Source: three-view drawing plus pictorial views. Frame: mm from the lowest corner of the part. A direction names the side the tool comes from. Give positions to 0.01 mm unless a question says otherwise; leave off trailing zeros. Loops run counter-clockwise (first coordinate to the right, second up) from the corner with the lowest first, then second, coordinate; pieces in that order, holes last. Notation, with made-up numbers: (-15.5, -14.5) -> (10.5, -14.5) arc R9 ccw to (10.5, 2.5) -> close; hole circle Ø6 at (75, 81). An arc over 180 degrees is marked (long way). Answer in a Markdown table with one row per item. Add a question column.
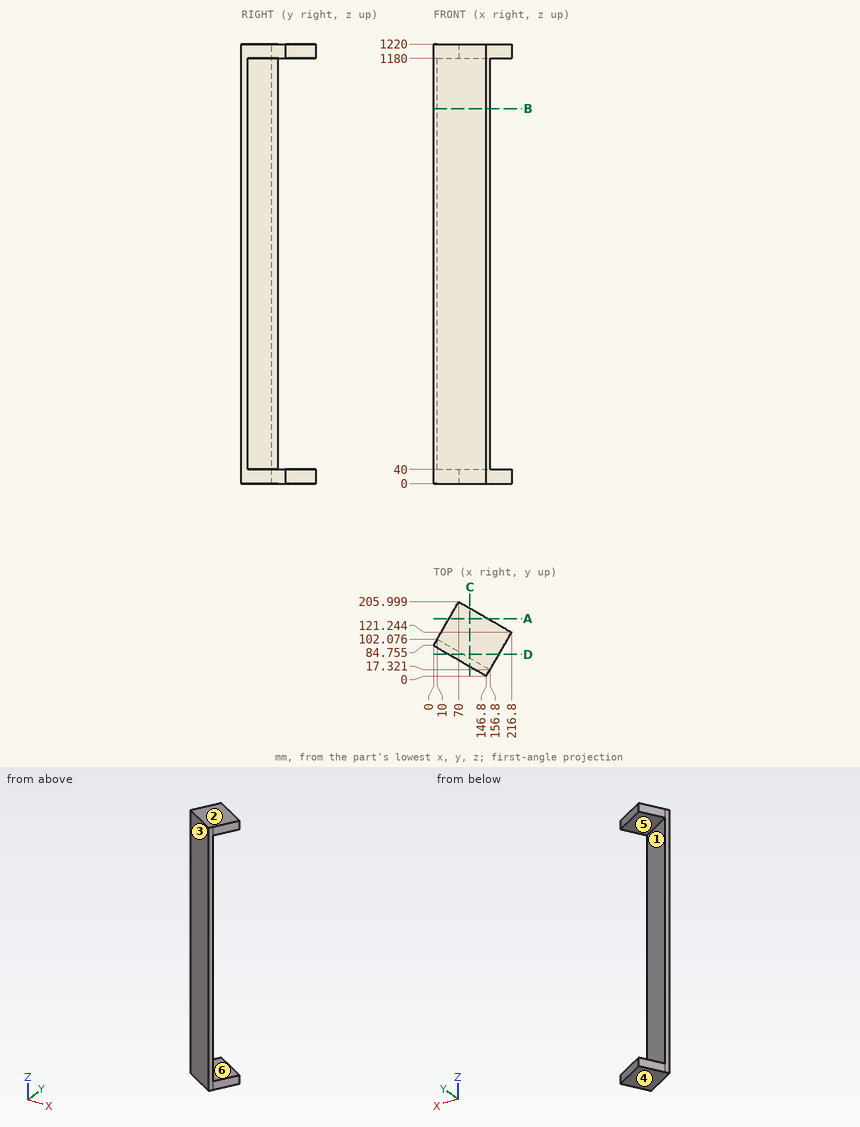
(1) Material intervals for line 1 along Z through (x, y) = (180, 99.5); line 2 along Y through (x, z) = (151, 1076.5) (1 decimal); line 3 along X through (y, z) = (12, 1018.5) (1 decimal), sorted ascending. Write a range as from..to.
(2) Cut plane D-D on y = 60. Return the cut outline in (x, z), then the cut area to 3 significant figures.
(3) Cut plane B-B on z = 1040.5. Return the cut outline in (x, y) (1 decimal), then the cut area to 3 significant figures.
(4) Cut plane A-A on y = 159. Return the cut outline in (x, z) (1 decimal).
(5) Draft query along Z for the marked faces 3, 4, 5 and 6. Return one class per face: +Z half, -Z half, draft (parallel to the pull), parting line (faces both ways), or undercut.
(6) Cut plane C-C on x = 100.5. Return the cut outline in (y, z) (1 decimal).
(7) Pin query (flat end, axial travel): pin 1 Ø1.5 at (x, z) = (54, 790.5) entering from -Y (1 decimal); pin 2 Ø4 at (x, z) = (123, 642.5) entering from -Y (1 decimal); pin 3 Ø10 at (x, z) = (122, 304) entering from +Y. Return the tip coordinate at first contact, or that it passes through.
(8) Reachability of the marked faces 1 and 2 from +Z, -Z, +X, -X, +Y, -Y: full face, straight path, thin tool, end or side. Return the list, or none.
Answer list:
| question | item | result |
|---|---|---|
| 1 | line 1 | z = 0..40, 1180..1220 |
| 1 | line 2 | y = 7.3..20.7 |
| 1 | line 3 | x = 126..153.7 |
| 2 | outline | (42.88, 0) -> (181.44, 0) -> (181.44, 40) -> (82.88, 40) -> (82.88, 1180) -> (181.44, 1180) -> (181.44, 1220) -> (42.88, 1220) -> close |
| 2 | area | 56,700 mm² |
| 3 | outline | (0, 84.8) -> (146.8, 0) -> (156.8, 17.3) -> (10, 102.1) -> close |
| 3 | area | 3,390 mm² |
| 4 | outline | (42.9, 0) -> (151.4, 0) -> (151.4, 40) -> (42.9, 40) -> close; (42.9, 1180) -> (151.4, 1180) -> (151.4, 1220) -> (42.9, 1220) -> close |
| 5 | face 3 | draft |
| 5 | face 4 | -Z half |
| 5 | face 5 | undercut |
| 5 | face 6 | undercut |
| 6 | outline | (26.7, 0) -> (188.4, 0) -> (188.4, 40) -> (49.8, 40) -> (49.8, 1180) -> (188.4, 1180) -> (188.4, 1220) -> (26.7, 1220) -> close |
| 7 | pin 1 | stops at y = 53.1 |
| 7 | pin 2 | stops at y = 12.6 |
| 7 | pin 3 | stops at y = 40.3 |
| 8 | face 1 | +X, +Y |
| 8 | face 2 | +Z, +X, -X, +Y, -Y |
